Check sheet for the drawn part. Datum: minimum x, y, z corner. Units: mm. A direction names the side the tool comes from. Give positions to 0.01 mm unless a question says otherwise; leave off trailing zeros. Order: outer loops, then holes, each group sorted by start corner. A loop starts at its lowest first (then second) coordinate and runs counter-clockwise, first axis right, second up. Notation, with made-up numbers: M -14.5,64.25 L 1.5,64.25 A29 cw 1.5,101.25 Z; hole C 54,31.5 d4. An arc over 180 degrees is marked long. Put each result on its own line as item: value. Start each with the question number.
Q1. Section check A-A on z = 70. Record the cut outline in (x, y).
Q2. Section check B-B on y = 22. Record the cut outline in (x, z), then the cut area to 3 significant figures.
Q3. Access from +Z, -Z, +X, -X, +Y, -Y to the whole of each face (thin tool, end or side, straight path). Record for the marked faces 1 and 2.
Q4. Material ranges on L1, parallel to Y at x = 46.5, z = 84.5; L2, parallel to Y at x = 10, z = 46, recorded low to high.
Q5. Go/stop test with flat-tipped pins: pin 1 (1 mm diameter, centred on x = 26.5, z = 15, fed in from +Y); pin 2 (10 mm diameter, centred on x = 14.5, y = 27, fed in from -Z); pin 3 (15.5 mm diameter, centred on y = 32, z = 47.5, fed in from +X). Record where each tip stops, or that it passes through.
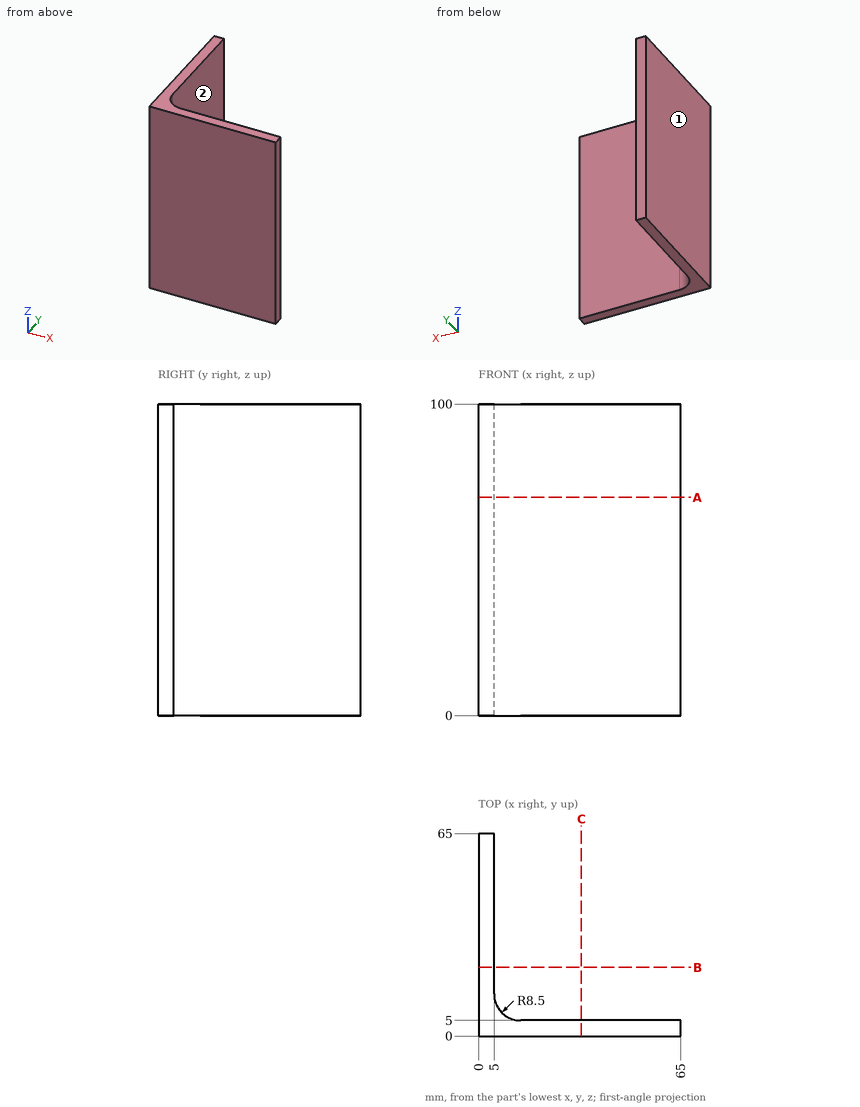
Results found:
1. outline: M 0,0 L 65,0 L 65,5 L 13.5,5 A8.5 cw 5,13.5 L 5,65 L 0,65 Z
2. outline: M 0,0 L 5,0 L 5,100 L 0,100 Z
2. area: 500 mm^2
3. face 1: +Z, -Z, -X, +Y, -Y
3. face 2: +Z, -Z, +X, +Y
4. L1: y = 0 to 5
4. L2: y = 0 to 5.75
5. pin 1: stops at y = 5
5. pin 2: passes through
5. pin 3: stops at x = 5
